Work out the finished part from the listing and answer in its coordinate system (mm). A direction names the side the tool comes from. Give positions to 0.01 mm unless a question says otherwise; leave off trailing zeros. Write each loop counter-clockwise with the first axis right and the second up, starting at its lowest first coordinate (ties: lowest second). Pieces come first, ordered by that corner, then holes. Notation, with made-up numbers: (62, 81.25) -> (88, 81.25) arc R14 ccw to (88, 102.25) -> close; hole circle Ø4 at (40, 52.25). An arc over 180 degrees is marked (long way). Use a Markdown table: item, result. Add a question column.
Q1. For faces 1 (the face through (11.1, -1, 22)), 2 (the face through (35, -3, 22)), 3 (the face through (17, 1, 34)), determine the directions among +Z, -Z, +X, -X, +Y, -Y from which every point of the face is accessible in a straight line to the end or side of a thin tool.
Q2. Each of these flat-tipped pins is pushed along its axis until it touches: pin 1 Ø0.9 at (x, z) = (13, 33) entering from +Y; pin 2 Ø2 at (x, y) = (12, -11.5) entering from +Z; pin 3 Ø9 at (x, z) = (14, 9) entering from +Y. Where does it stop, or does it pass through?
Q3. For a pull along Z with two mould halves and no side action, classify faces 4 (the face through (21, -20, 29)), 5 (the face through (28.986, -9.86, 32.535)), 6 (the face through (0, 3, 17)) as pulls with the +Z half, pulls with the -Z half, needs draft (parallel to the pull), parting line crosses it, or undercut.
Q4. Section C-C, the plane y = 3.5 is taken. State how many separate pieces and enclosed holes the cut face has, plus the area to 3 significant figures.
Q5. Section A-A, the plane z = 1 is taken. Give the vertices of the cut face in (x, y).
Q6. Consider line 1 (X direction, y = 3.85, z = 1); line 2 (X direction, y = 2.85, z = 32.45); line 3 (Z direction, x = 23.5, y = 1.25). Determine where each line is inside the solid, lowest interval first.
from build123d import *

# Parameters (mm, degrees)
BOSS_EXTRU_1_DEPTH       = 35
ENL_V_MAT_EXTRU_1_DEPTH  = 3
ENL_V_START              = -2
ESQUISSE3_W              = 14
ESQUISSE3_H              = 12
ENL_V_MAT_EXTRU_2_DEPTH  = 2
ESQUISSE7_W              = 3
ESQUISSE7_H              = 12
ENL_V_MAT_EXTRU_4_DEPTH  = 2
BOSS_EXTRU_4_START       = -2
ESQUISSE9_W              = 1.1
ESQUISSE9_H              = 12
BOSS_EXTRU_4_DEPTH       = 2
ESQUISSE10_R             = 0.8
BOSS_EXTRU_5_DEPTH       = 6.285817
ESQUISSE19_W             = 2
ESQUISSE19_H             = 4.092832792
ESQUISSE19_H_2           = 4.443065592
ESQUISSE19_W_2           = 4
ESQUISSE19_H_3           = 2
BOSS_EXTRU_8_DEPTH       = 6.285817
ENL_V_MAT_EXTRU_9_DEPTH  = 2
ESQUISSE25_R             = 0.8
BOSS_EXTRU_10_DEPTH      = 5
ESQUISSE26_R             = 0.8
BOSS_EXTRU_11_DEPTH      = 5
ESQUISSE27_R             = 0.8
BOSS_EXTRU_12_DEPTH      = 5
ESQUISSE28_R             = 2.55
ESQUISSE28_R_2           = 0.8
BOSS_EXTRU_13_DEPTH      = 6.290743
ENL_V_START_2            = -6.290743
ESQUISSE29_W             = 1.350487441
ESQUISSE29_H             = 4.654500935
ENL_V_MAT_EXTRU_11_DEPTH = 6.290743
BOSS_EXTRU_14_DEPTH      = 20
ENL_V_START_3            = -17.727203
ENL_V_MAT_EXTRU_12_DEPTH = 17.727203


with BuildPart() as part:
    # Esquisse1 → Boss.-Extru.1 (new body)
    with BuildSketch(Plane.XY):
        Polygon((0, 0), (34, 0), (34, 5), (32, 5), (32, 2), (2, 2), (2, 5), (0, 5), align=None)
    extrude(amount=BOSS_EXTRU_1_DEPTH)

    # Esquisse2 → Enl_v. mat.-Extru.1 (cut)
    with BuildSketch(Plane.XY.offset(35)):
        Polygon((2, 5), (1, 5), (1, 1), (33, 1), (33, 5), (32, 5), (32, 2), (2, 2), align=None)
    extrude(amount=-ENL_V_MAT_EXTRU_1_DEPTH, mode=Mode.SUBTRACT)

    # Esquisse3 → Enl_v. mat.-Extru.2 (cut)
    with BuildSketch(Plane(origin=(0, 2, 0), x_dir=(1, 0, 0), z_dir=(0, 1, 0)).offset(ENL_V_START)):
        with Locations((17, -22)):
            Rectangle(ESQUISSE3_W, ESQUISSE3_H)
    extrude(amount=ENL_V_MAT_EXTRU_2_DEPTH, mode=Mode.SUBTRACT)

    # Esquisse7 → Enl_v. mat.-Extru.4 (cut)
    with BuildSketch(Plane.XZ.offset(ENL_V_START)):
        with Locations((25.5, 22)):
            Rectangle(ESQUISSE7_W, ESQUISSE7_H)
    extrude(amount=ENL_V_MAT_EXTRU_4_DEPTH, mode=Mode.SUBTRACT)

    # Esquisse9 → Boss.-Extru.4 (add)
    with BuildSketch(Plane.XZ.offset(BOSS_EXTRU_4_START)):
        with Locations((10.55, 22)):
            Rectangle(ESQUISSE9_W, ESQUISSE9_H)
    extrude(amount=BOSS_EXTRU_4_DEPTH)

    # Esquisse10 → Boss.-Extru.5 (add)
    with BuildSketch(Plane.XZ):
        with BuildLine():
            Line((11.1, 22.988338073), (11.1, 21.361894727))
            ThreePointArc((11.1, 21.361894727), (7.27279708, 22.1751164), (11.1, 22.988338073))
        make_face()
        with Locations(Location((9.27279708, 22.1751164, 0), (0, 0, 90))):
            Circle(ESQUISSE10_R, mode=Mode.SUBTRACT)
    extrude(amount=BOSS_EXTRU_5_DEPTH)

    # Esquisse19 → Boss.-Extru.8 (add)
    with BuildSketch(Plane.XZ):
        with Locations((9.27279708, 25.953583604)):
            Rectangle(ESQUISSE19_W, ESQUISSE19_H)
        with Locations((9.27279708, 18.221532796)):
            Rectangle(ESQUISSE19_W, ESQUISSE19_H_2)
        with Locations((5.540746272, 22.1751164)):
            Rectangle(ESQUISSE19_W_2, ESQUISSE19_H_3)
    extrude(amount=BOSS_EXTRU_8_DEPTH)

    # Esquisse21 → Enl_v. mat.-Extru.9 (cut)
    with BuildSketch(Plane(origin=(0, 0, 21.1751164), x_dir=(-1, 0, 0), z_dir=(0, 0, -1))):
        Polygon((-3.540746272, 0), (-7.540746272, -6.285817331), (-3.540746272, -6.285817331), align=None)
    extrude(amount=-ENL_V_MAT_EXTRU_9_DEPTH, mode=Mode.SUBTRACT)

    # Esquisse25 → Boss.-Extru.10 (add)
    with BuildSketch(Plane.XZ):
        with BuildLine():
            Line((0, 31.45), (-1, 31.45))
            ThreePointArc((-1, 31.45), (-5.895740821, 32.45), (-1, 33.45))
            Line((-1, 33.45), (0, 33.45))
            Line((0, 33.45), (0, 31.45))
        make_face()
        with Locations(Location((-3.345740821, 32.45, 0), (0, 0, 270))):
            Circle(ESQUISSE25_R, mode=Mode.SUBTRACT)
        with BuildLine():
            Line((34, 33.45), (35, 33.45))
            ThreePointArc((35, 33.45), (39.895740821, 32.45), (35, 31.45))
            Line((35, 31.45), (34, 31.45))
            Line((34, 31.45), (34, 33.45))
        make_face()
        with Locations(Location((37.345740821, 32.45, 0), (0, 0, 90))):
            Circle(ESQUISSE25_R, mode=Mode.SUBTRACT)
    extrude(amount=-BOSS_EXTRU_10_DEPTH)

    # Esquisse26 → Boss.-Extru.11 (add)
    with BuildSketch(Plane.XZ):
        with BuildLine():
            Line((-1, 2), (0, 2))
            Line((0, 2), (0, 0))
            Line((0, 0), (-1, 0))
            ThreePointArc((-1, 0), (-5.895740821, 1), (-1, 2))
        make_face()
        with Locations(Location((-3.345740821, 1, 0), (0, 0, 270))):
            Circle(ESQUISSE26_R, mode=Mode.SUBTRACT)
        with BuildLine():
            Line((34, 2), (34, 0))
            Line((34, 0), (35, 0))
            ThreePointArc((35, 0), (39.895740821, 1), (35, 2))
            Line((35, 2), (34, 2))
        make_face()
        with Locations(Location((37.345740821, 1, 0), (0, 0, 90))):
            Circle(ESQUISSE26_R, mode=Mode.SUBTRACT)
    extrude(amount=-BOSS_EXTRU_11_DEPTH)

    # Esquisse27 → Boss.-Extru.12 (add)
    with BuildSketch(Plane(origin=(0, 0, 0), x_dir=(-1, 0, 0), z_dir=(0, -1, 0))):
        with BuildLine():
            Line((-34, -21.1751164), (-34.527056259, -21.1751164))
            ThreePointArc((-34.527056259, -21.1751164), (-39.42279708, -22.1751164), (-34.527056259, -23.1751164))
            Line((-34.527056259, -23.1751164), (-34, -23.1751164))
            Line((-34, -23.1751164), (-34, -21.1751164))
        make_face()
        with Locations(Location((-36.87279708, -22.1751164, 0), (0, 0, 90))):
            Circle(ESQUISSE27_R, mode=Mode.SUBTRACT)
    extrude(amount=-BOSS_EXTRU_12_DEPTH)

    # Esquisse28 → Boss.-Extru.13 (add)
    with BuildSketch(Plane.XZ):
        with Locations(Location((36.87279708, 22.1751164, 0), (0, 0, 270))):
            Circle(ESQUISSE28_R)
        with Locations(Location((36.87279708, 22.1751164, 0), (0, 0, 270))):
            Circle(ESQUISSE28_R_2, mode=Mode.SUBTRACT)
    extrude(amount=BOSS_EXTRU_13_DEPTH)

    # Esquisse29 → Enl_v. mat.-Extru.11 (cut)
    with BuildSketch(Plane.XZ.offset(6.290743087).offset(ENL_V_START_2)):
        with Locations((34.324427693, 22.303512705)):
            Rectangle(ESQUISSE29_W, ESQUISSE29_H)
    extrude(amount=ENL_V_MAT_EXTRU_11_DEPTH, mode=Mode.SUBTRACT)

    # Esquisse30 → Boss.-Extru.14 (add)
    with BuildSketch(Plane.XZ):
        Polygon((8.27279708, 28), (34, 28), (34, 30), (30, 30), (30, 35), (28, 35), (28, 30), (22.16279708, 30), (22.16279708, 35), (20.16279708, 35), (20.16279708, 30), (14.27279708, 30), (14.27279708, 35), (12.27279708, 35), (12.27279708, 30), (8.27279708, 30), align=None)
        Polygon((8.27279708, 16), (34, 16), (34, 14), (30, 14), (30, 9), (28, 9), (28, 14), (22.11, 14), (22.11, 9), (20.11, 9), (20.11, 14), (14.27279708, 14), (14.27279708, 9), (12.27279708, 9), (12.27279708, 14), (8.27279708, 14), align=None)
    extrude(amount=BOSS_EXTRU_14_DEPTH)

    # Esquisse31 → Enl_v. mat.-Extru.12 (cut)
    with BuildSketch(Plane(origin=(30, 0, 0), x_dir=(0, 0, -1), z_dir=(1, 0, 0)).offset(ENL_V_START_3)):
        Polygon((-35, 0), (-30, -20), (-35, -20), align=None)
        Polygon((-9, 0), (-14, -20), (-9, -20), align=None)
    extrude(amount=ENL_V_MAT_EXTRU_12_DEPTH, mode=Mode.SUBTRACT)


solid = part.part
Result set:
| question | item | result |
|---|---|---|
| 1 | face 1 | +Y, -Y |
| 1 | face 2 | +Z, -Z, -Y |
| 1 | face 3 | +Z, +Y |
| 2 | pin 1 | stops at y = 1 |
| 2 | pin 2 | stops at z = 32.37 |
| 2 | pin 3 | stops at y = 2 |
| 3 | face 4 | needs draft |
| 3 | face 5 | pulls with the +Z half |
| 3 | face 6 | undercut |
| 4 | separate pieces | 2 |
| 4 | enclosed holes | 5 |
| 4 | area | 234 mm2 |
| 5 | outline | (-5.9, 0) -> (-4.15, 0) -> (-4.15, 5) -> (-5.9, 5) -> close; (-2.55, 0) -> (36.55, 0) -> (36.55, 5) -> (32, 5) -> (32, 2) -> (2, 2) -> (2, 5) -> (-2.55, 5) -> close; (38.15, 0) -> (39.9, 0) -> (39.9, 5) -> (38.15, 5) -> close |
| 6 | line 1 | x = -5.9 to -4.15, -2.55 to 2, 32 to 36.55, 38.15 to 39.9 |
| 6 | line 2 | x = -5.9 to -4.15, -2.55 to 1, 33 to 36.55, 38.15 to 39.9 |
| 6 | line 3 | z = 0 to 16, 28 to 32 |
